Study the drawing (mm; zero at the part's minimum x, y, z) and answer. A direction names the side the tool comes from. Give positions to 0.01 mm unless a question says otherwise; leave off trailing zeros. Write each loop counter-clockwise with the first axis right and the second up, starting at its lowest first coordinate (ties: lowest second). Pieces come first, ordered by that corner, then holes. Notation, with made-up numbers: M 49,-7 L 75,-7 A10 ccw 75,0 Z; hole C 80.5,29.25 d11. An arc over 180 degrees is marked long. Use a Markdown table: item, result. Add a question column.
Item 1: A cutting plane is placed at A-A on x = 11.5. Determine the outline of the cut face in (y, z), then the cut area to 3 significant figures.
Item 2: A cutting plane is placed at D-D on y = 15. Determine the outline of the cut face in (x, z), then the cut area to 3 significant figures.
Item 3: Given P1, Ø8, axis at x = 11.5, y = 6, coming from the -Z side; P2, Ø1.8, axis at x = 4, z = 4, coming from the +Y side; P3, Ø2, axis at x = 2.5, z = 3.5, coming from the -Y side; P4, Ø2, axis at x = 15, y = 13.5, coming from the -Z side, each flat-ended and moving along its own axis, determine where each tip first touches the part or whether it passes through.
Item 4: A cutting plane is placed at C-C on y = 6. Determine the outline of the cut face in (x, z), then the cut area to 3 significant figures.
Item 5: For the marked faces 1, 2 and 3, determine the directions among +Z, -Z, +X, -X, +Y, -Y from which every point of the face is accessible in a straight line to the end or side of a thin tool.
Item 6: A cutting plane is placed at B-B on z = 11. Determine the outline of the cut face in (x, y), then the cut area to 3 significant figures.
Item 7: Consider probe 1 along X at (y, z) = (14.5, 4); probe 2 along Y at (x, z) = (11.5, 12.5); probe 3 along Z at (x, y) = (4, 14). Determine where each line is inside the solid, lowest interval first. Write a range as [from, to].
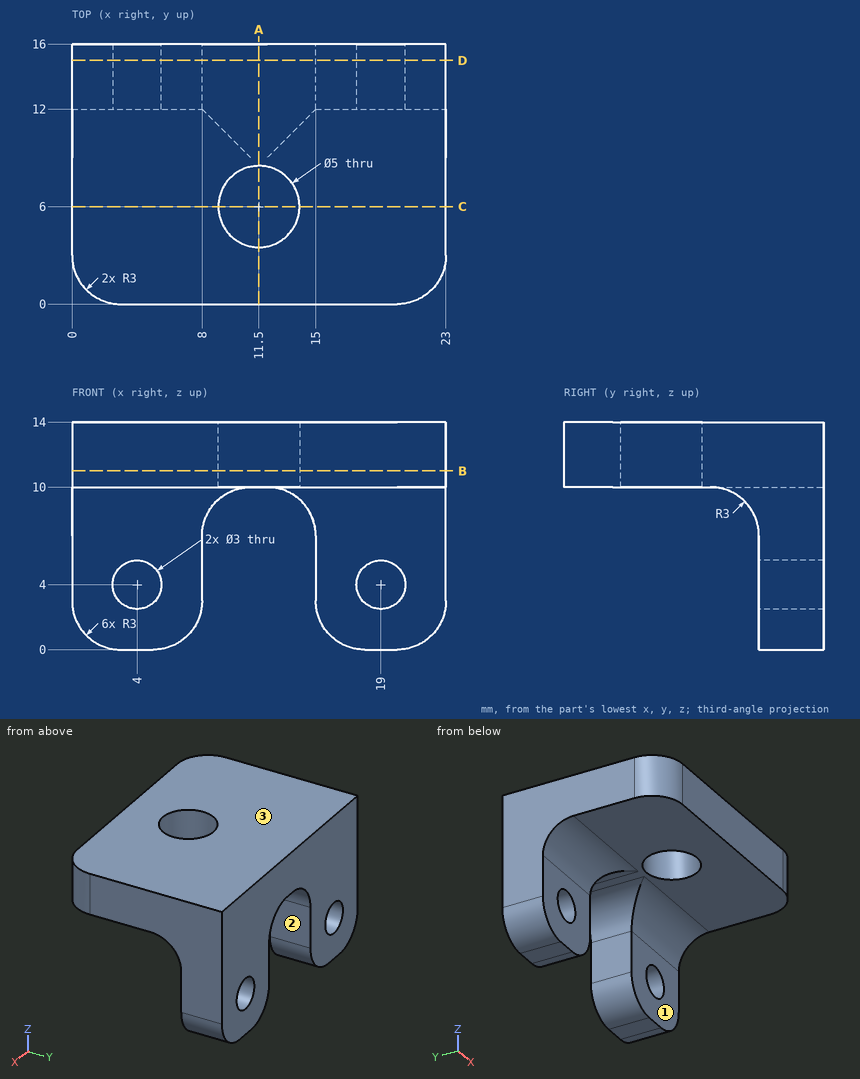
Filled in:
| question | item | result |
|---|---|---|
| 1 | outline | M 0,10 L 3.5,10 L 3.5,14 L 0,14 Z; M 8.5,10 L 16,10 L 16,14 L 8.5,14 Z |
| 1 | area | 44.0 mm² |
| 2 | outline | M 0,3 A3 ccw 3,0 L 5,0 A3 ccw 8,3 L 8,7 A3 cw 11,10 L 12,10 A3 cw 15,7 L 15,3 A3 ccw 18,0 L 20,0 A3 ccw 23,3 L 23,14 L 0,14 Z; hole C 4,4 d3; hole C 19,4 d3 |
| 2 | area | 234 mm² |
| 3 | P1 | z = 9.89 |
| 3 | P2 | through |
| 3 | P3 | y = 12 |
| 3 | P4 | z = 0.76 |
| 4 | outline | M 0,10 L 9,10 L 9,14 L 0,14 Z; M 14,10 L 23,10 L 23,14 L 14,14 Z |
| 4 | area | 72.0 mm² |
| 5 | face 1 | -Z, +X, -X, -Y |
| 5 | face 2 | -Z, +Y, -Y |
| 5 | face 3 | +Z, +X, -X, +Y, -Y |
| 6 | outline | M 0,3 A3 ccw 3,0 L 20,0 A3 ccw 23,3 L 23,16 L 0,16 Z; hole C 11.5,6 d5 |
| 6 | area | 345 mm² |
| 7 | probe 1 | [0, 2.5], [5.5, 8], [15, 17.5], [20.5, 23] |
| 7 | probe 2 | [0, 3.5], [8.5, 16] |
| 7 | probe 3 | [0, 2.5], [5.5, 14] |
